For this review, take the finished solid that the model builds, in its own axes (mm). Round coordinates to 2 decimals unless told otherwise and drop trailing zeros. Order: outer loops, then holes, each group sorted by start corner. A loop starts at its lowest first (then second) coordinate and runs counter-clockwise, first axis right, second up. Notation, with made-up numbers: M 28.25,24.25 L 52.25,24.25 A14 ccw 52.25,40.25 Z; hole C -11.5,80 d1. An arc over 180 degrees is marked long. Answer in a Markdown table with one row per item. Add a question column.
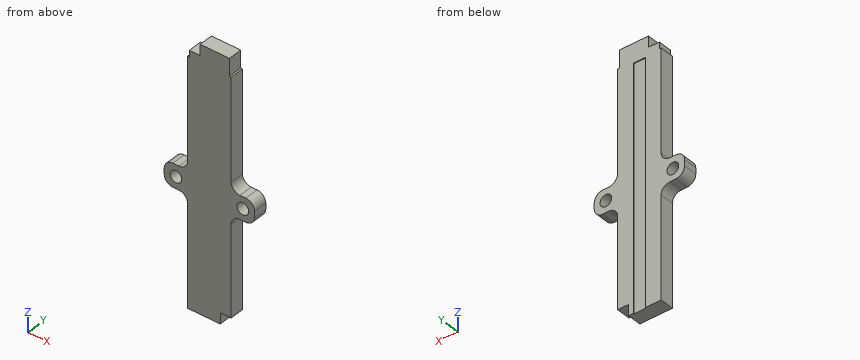
```python
from build123d import *

# Parameters (mm, degrees)
SKETCH1_W               = 12.7
SKETCH1_H               = 4.064
BOSS_EXTRUDE1_DEPTH     = 228.6
SKETCH2_W               = 3.429
SKETCH2_H               = 217.3732
CUT_EXTRUDE1_DEPTH      = 0.254
SKETCH3_W               = 0.508
SKETCH3_H               = 5.08
CUT_EXTRUDE2_DEPTH      = 229.724285103
MIRROR2_COPY_1_SKETCH_W = 0.508
MIRROR2_COPY_1_SKETCH_H = 5.08
MIRROR2_COPY_1_DEPTH    = 229.724285103
SKETCH4_W               = 3.175
SKETCH4_H               = 3.175
CUT_EXTRUDE3_DEPTH      = 229.724285103
CUT_EXTRUDE4_DEPTH      = 229.724285103
SKETCH7_W               = 6.80212
SKETCH7_H               = 6.80212
SKETCH7_R               = 1.70053
BOSS_EXTRUDE2_DEPTH     = 4.064
FILLET1_R               = 2.54


with BuildPart() as part:
    # Sketch1 → Boss-Extrude1 (new body)
    with BuildSketch(Plane.XY):
        Rectangle(SKETCH1_W, SKETCH1_H)
    extrude(amount=BOSS_EXTRUDE1_DEPTH)

    # Sketch2 → Cut-Extrude1 (cut)
    with BuildSketch(Plane(origin=(0, 2.032, 0), x_dir=(1, 0, 0), z_dir=(0, 1, 0))):
        with Locations((0, -114.3)):
            Rectangle(SKETCH2_W, SKETCH2_H)
    extrude(amount=-CUT_EXTRUDE1_DEPTH, mode=Mode.SUBTRACT)

    # Sketch3 → Cut-Extrude2 (cut, through all)
    with BuildSketch(Plane(origin=(0, 2.032, 0), x_dir=(1, 0, 0), z_dir=(0, 1, 0))):
        with Locations((-6.096, -226.06)):
            Rectangle(SKETCH3_W, SKETCH3_H)
    cut_extrude2 = extrude(amount=-CUT_EXTRUDE2_DEPTH, mode=Mode.SUBTRACT)

    # Mirror1: Cut-Extrude2 across plane
    add(cut_extrude2.mirror(Plane(origin=(0, 0, 114.3), x_dir=(1, 0, 0), z_dir=(0, 0, -1))), mode=Mode.SUBTRACT)

    # Mirror2: Cut-Extrude2 across plane
    add(cut_extrude2.mirror(Plane(origin=(0, 0, 0), x_dir=(0, 0, 1), z_dir=(1, 0, 0))), mode=Mode.SUBTRACT)

    # Mirror2 copy 1 sketch → Mirror2 copy 1 (cut, through all)
    with BuildSketch(Plane(origin=(0, 2.032, 228.6), x_dir=(-1, 0, 0), z_dir=(0, 1, 0))):
        with Locations((-6.096, -226.06)):
            Rectangle(MIRROR2_COPY_1_SKETCH_W, MIRROR2_COPY_1_SKETCH_H)
    extrude(amount=-MIRROR2_COPY_1_DEPTH, mode=Mode.SUBTRACT)

    # Sketch4 → Cut-Extrude3 (cut, through all)
    with BuildSketch(Plane(origin=(0, 2.032, 0), x_dir=(1, 0, 0), z_dir=(0, 1, 0))):
        with Locations((-4.2545, -227.0125)):
            Rectangle(SKETCH4_W, SKETCH4_H)
    extrude(amount=-CUT_EXTRUDE3_DEPTH, mode=Mode.SUBTRACT)

    # Sketch5 → Cut-Extrude4 (cut, through all)
    with BuildSketch(Plane(origin=(0, 2.032, 0), x_dir=(1, 0, 0), z_dir=(0, 1, 0))):
        Polygon((-6.35, 0), (6.35, 0), (6.35, -152.4), (6.35, -155.575), (3.175, -155.575), (3.175, -152.4), (-6.35, -152.4), align=None)
    extrude(amount=-CUT_EXTRUDE4_DEPTH, mode=Mode.SUBTRACT)

    # Sketch7 → Boss-Extrude2 (add, through all)
    # profile 1 of 2: a face of its own
    with BuildSketch(Plane(origin=(0, 2.032, 0), x_dir=(1, 0, 0), z_dir=(0, 1, 0))):
        with Locations((9.75106, -187.96)):
            Rectangle(SKETCH7_W, SKETCH7_H)
        with Locations(Location((9.75106, -187.96, 0), (0, 0, 270))):
            Circle(SKETCH7_R, mode=Mode.SUBTRACT)
    # profile 2 of 2: a face of its own
    with BuildSketch(Plane(origin=(0, 2.032, 0), x_dir=(1, 0, 0), z_dir=(0, 1, 0))):
        with Locations((-9.75106, -187.96)):
            Rectangle(SKETCH7_W, SKETCH7_H)
        with Locations(Location((-9.75106, -187.96, 0), (0, 0, 270))):
            Circle(SKETCH7_R, mode=Mode.SUBTRACT)
    extrude(amount=-BOSS_EXTRUDE2_DEPTH)

    # Fillet1
    fillet1_edges = [part.edges().sort_by_distance(p)[0] for p in [
        (6.35, 0, 191.36106),
        (13.15212, 0, 191.36106),
        (13.15212, 0, 184.55894),
        (6.35, 0, 184.55894),
        (-13.15212, 0, 184.55894),
        (-6.35, 0, 184.55894),
        (-13.15212, 0, 191.36106),
        (-6.35, 0, 191.36106),
    ]]
    fillet(fillet1_edges, radius=FILLET1_R)


solid = part.part
```
1. Consider section B-B on y = -0.95. State how many separate pieces and enclosed holes the cut face has, plus the area to 3 significant figures.
2. Consider section A-A on z = 187.96. Write out the cut boundary in (x, y).
3. Consider section D-D on x = 7.25. Write out the cut boundary in (y, z), plus the area to 3 significant figures.
4. Clearance check with flat-ended pins moving along their axes: pin 1 Ø0.9 at (x, y) = (10, 0.5) entering from +Z; pin 2 Ø1 at (x, y) = (-4, 0.5) entering from +Z (3 decimals); pin 3 Ø2 at (y, z) = (-0.5, 173.5) entering from +X. State where each tip first meets the part, or that it passes through.
5. To check wall thickness, follow probe 1 along X at (y, z) = (0.35, 187.96); probe 2 along Z at (x, y) = (-6, -1.5); probe 3 along Y at (x, z) = (0, 213). State the ranges of each line that lie inside material, in increasing order. Write a range as [from, to].
6. Consider section C-C on z = 161.5. Write out the cut boundary in (x, y).
Solved:
| question | item | result |
|---|---|---|
| 1 | separate pieces | 1 |
| 1 | enclosed holes | 2 |
| 1 | area | 1,020 mm^2 |
| 2 | outline | M -13.15,-2.03 L -11.45,-2.03 L -11.45,2.03 L -13.15,2.03 Z; M -8.05,-2.03 L 8.05,-2.03 L 8.05,2.03 L 1.71,2.03 L 1.71,1.78 L -1.71,1.78 L -1.71,2.03 L -8.05,2.03 Z; M 11.45,-2.03 L 13.15,-2.03 L 13.15,2.03 L 11.45,2.03 Z |
| 3 | outline | M -2.03,183.96 L 2.03,183.96 L 2.03,191.96 L -2.03,191.96 Z |
| 3 | area | 32.5 mm^2 |
| 4 | pin 1 | stops at z = 191.36 |
| 4 | pin 2 | stops at z = 225.425 |
| 4 | pin 3 | stops at x = 6.35 |
| 5 | probe 1 | x = [-13.15, -11.45], [-8.05, 8.05], [11.45, 13.15] |
| 5 | probe 2 | z = [152.4, 223.52] |
| 5 | probe 3 | y = [-2.03, 1.78] |
| 6 | outline | M -6.35,-2.03 L 6.35,-2.03 L 6.35,2.03 L 1.71,2.03 L 1.71,1.78 L -1.71,1.78 L -1.71,2.03 L -6.35,2.03 Z |
